CAD build for the part. Positions are in the model's coordinates, mm. A direction names the side the tool comes from. Round coordinates to 2 decimals unless told otherwise and drop trailing zeros. Loops run counter-clockwise (first coordinate to the right, second up) from the corner with the lowest first, then second, coordinate; pieces in that order, holes last. Notation, with made-up numbers: M 87.5,82 L 107.5,82 A35 ccw 107.5,118 Z; hole C 21,43.25 d5. An arc over 180 degrees is marked long. Use a Markdown table: item, result. Add a question column.
(1) Band-saw the part on C-C, the plane y = 4. Write the cut outline in (x, z).
(2) Which spindle directions (+Z, -Z, +X, -X, +Y, -Y) get a long thin tool onto all of the face, cutting with end or side? Do faces 1 (the face through (-0.54, 3.56, 2.44)), 2 (the face through (-2.9, 0.5, -0.1)). Say none if no direction does.
(3) Band-saw the part on A-A, the plane x = 0. Write the cut outline in (y, z).
(4) Band-saw the part on B-B, the plane z = 0. Write the cut outline in (x, y).
(5) Flat gauge pins, fed straight in: P1, Ø3, axis at y = 4.5, z = 2, coming from the -X side; P2, Ø3, axis at x = -1, z = 2, coming from the +Y side; P3, Ø3, axis at x = -1, z = 0, coming from the -Y side; P4, Ø1, axis at x = 2, z = 0.5, coming from the +Y side. Where does each tip first touch, or does it go through?
(6) Band-saw the part on D-D, the plane z = -1.55. Write the cut outline in (x, y), and give its area (3 significant figures).
(7) Wall check: L1, parallel to Z at x = -0.1, y = 2; L2, parallel to Y at x = -2.5, z = 0.9; L3, parallel to Y at x = -0.45, z = -2.2. Give the ranges that are in metal, low to high.
from build123d import *

# Parameters (mm, degrees)
SKETCH3_R           = 0.25
BOSS_EXTRUDE2_DEPTH = 3.2


with BuildPart() as part:
    # Sketch2 → Revolve1 (revolve)
    with BuildSketch(Plane.XY):
        with BuildLine():
            Line((2.5, 6.2), (2.5, 1))
            Line((2.5, 1), (2.9, 1))
            Line((2.9, 1), (2.9, 0))
            Line((2.9, 0), (0, 0))
            Line((0, 0), (0, 8.7))
            ThreePointArc((0, 8.7), (1.767766953, 7.967766953), (2.5, 6.2))
        make_face()
    revolve(axis=Axis((0, 0, 0), (0, 1, 0)))

    # Sketch3 → Boss-Extrude2 (add)
    with BuildSketch(Plane(origin=(0, 0, 0), x_dir=(1, 0, 0), z_dir=(0, 1, 0))):
        with Locations((-1.27, 0)):
            Circle(SKETCH3_R)
        with Locations((1.27, 0)):
            Circle(SKETCH3_R)
    extrude(amount=-BOSS_EXTRUDE2_DEPTH)


solid = part.part
Return value:
| question | item | result |
|---|---|---|
| 1 | outline | C 0,0 d5 |
| 2 | face 1 | +Y |
| 2 | face 2 | +Y, -Y |
| 3 | outline | M 0,-2.9 L 1,-2.9 L 1,-2.5 L 6.2,-2.5 A2.5 ccw 6.2,2.5 L 1,2.5 L 1,2.9 L 0,2.9 Z |
| 4 | outline | M -2.9,0 L -1.52,0 L -1.52,-3.2 L -1.02,-3.2 L -1.02,0 L 1.02,0 L 1.02,-3.2 L 1.52,-3.2 L 1.52,0 L 2.9,0 L 2.9,1 L 2.5,1 L 2.5,6.2 A2.5 ccw -2.5,6.2 L -2.5,1 L -2.9,1 Z |
| 5 | P1 | x = -2.45 |
| 5 | P2 | y = 8.59 |
| 5 | P3 | y = -3.2 |
| 5 | P4 | y = 8.15 |
| 6 | outline | M -2.45,0 L 2.45,0 L 2.45,1 L 1.96,1 L 1.96,6.2 A1.96 ccw -1.96,6.2 L -1.96,1 L -2.45,1 Z |
| 6 | area | 31.3 mm^2 |
| 7 | L1 | -2.5 to 2.5 |
| 7 | L2 | 0 to 1 |
| 7 | L3 | 0 to 7.3 |
